Geometry check sheet. Reference: drawing and pictorial views, mm from the part's lowest x, y, z. Give positions to 0.01 mm unless a question says otherwise; leave off trailing zeros. Loops run counter-clockwise (first coordinate to the right, second up) from the corner with the lowest first, then second, coordinate; pieces in that order, holes last. Notation, with made-up numbers: (30, 69.5) - (47, 69.5) arc R7 cw to (47, 79.5) - close; hole circle Ø4 at (41, 73.25). An arc over 180 degrees is marked (long way). Use CSV: the item, a comma, the result in double quotes.
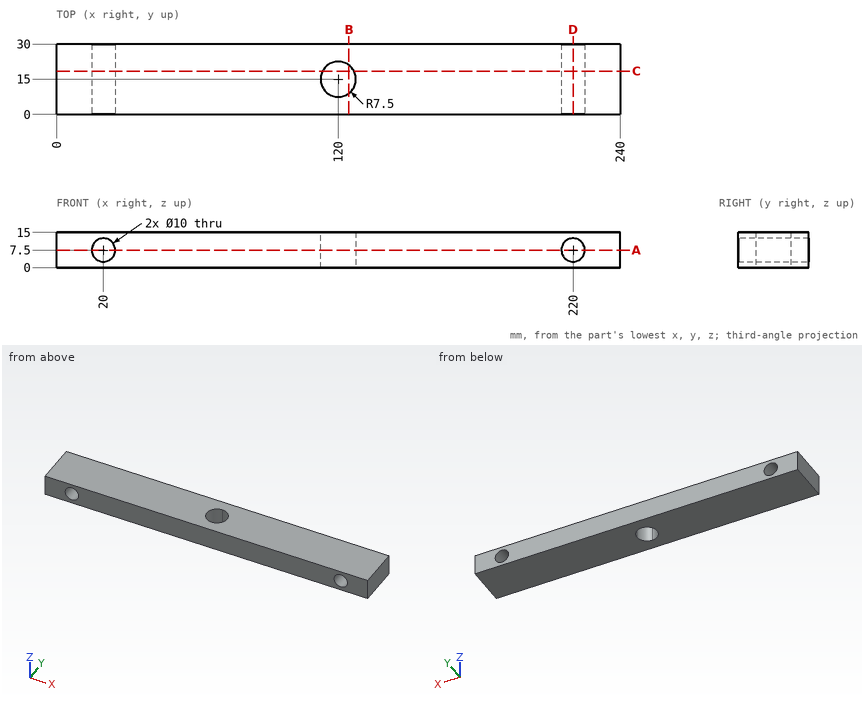
1. Sectioned sample at B-B, the plane x = 124.5. Record the boundary of the cut face in (y, z), and give its area (3 significant figures).
Completed:
outline,"(0, 0) - (9, 0) - (9, 15) - (0, 15) - close; (21, 0) - (30, 0) - (30, 15) - (21, 15) - close"
area,"270 mm²"
2. Sectioned sample at C-C, the plane y = 18.5. Record the boundary of the cut face in (x, z).
Completed:
outline,"(0, 0) - (113.37, 0) - (113.37, 15) - (0, 15) - close; (126.63, 0) - (240, 0) - (240, 15) - (126.63, 15) - close; hole circle Ø10 at (20, 7.5); hole circle Ø10 at (220, 7.5)"
3. Scan lines: line 1 along X through (y, z) = (15.25, 7.5); line 2 along X through (y, z) = (24.5, 9.25); line 3 along Z through (x, y) = (220, 25.25). Record each from-to range of solid material in increasing order.
Completed:
line 1,"x = 0 to 15, 25 to 112.5, 127.5 to 215, 225 to 240"
line 2,"x = 0 to 15.32, 24.68 to 215.32, 224.68 to 240"
line 3,"z = 0 to 2.5, 12.5 to 15"
4. Sectioned sample at D-D, the plane x = 220. Record the boundary of the cut face in (y, z), and give its area (3 significant figures).
Completed:
outline,"(0, 0) - (30, 0) - (30, 2.5) - (0, 2.5) - close; (0, 12.5) - (30, 12.5) - (30, 15) - (0, 15) - close"
area,"150 mm²"
5. Sectioned sample at A-A, the plane z = 7.5. Record the boundary of the cut face in (x, y).
Completed:
outline,"(0, 0) - (15, 0) - (15, 30) - (0, 30) - close; (25, 0) - (215, 0) - (215, 30) - (25, 30) - close; (225, 0) - (240, 0) - (240, 30) - (225, 30) - close; hole circle Ø15 at (120, 15)"
